Source: three-view drawing plus pictorial views. Frame: mm from the lowest corner of the part. Give positions to 0.01 mm unless a question says otherwise; leave off trailing zeros. Loops run counter-clockwise (first coordinate to the right, second up) from the corner with the lowest first, then second, coordinate; pieces in that order, holes last. Notation, with made-up numbers: M 41.25,-7 L 72.25,-7 A29 ccw 72.25,28 Z; hole C 29,-31 d2. An arc over 180 degrees is marked long. Answer as a JSON object with one key per item and string values. Group by question number.
1) Ray query, L1, parallel to X at y = 7, z = 147; L2, parallel to X at y = 18, z = 302 (1 decimal); L3, parallel to Z at x = 38.5, y = 15 (1 decimal). Return the intervals inside material, ascending.
2) Section query C-C on x = 79. Return loops of the section in (y, z).
3) Section query A-A on y = 14.5. Count the separate pieces of the cut face and the enclosed holes in it, plus the area to 3 significant figures.
4) First-contact query: P1, Ø9.5, axis at y = 13.5, z = 12.5, coming from the -X side; P2, Ø6, axis at x = 92.5, y = 11, coming from the -Z side; P3, Ø9.5, axis at y = 10, z = 10, coming from the +X side. Flat tips, straight axial feed; report the tip coordinate or a pass-through.
5) Section query B-B on z = 141. Return loops of the section in (x, y), plus the area to 3 significant figures.
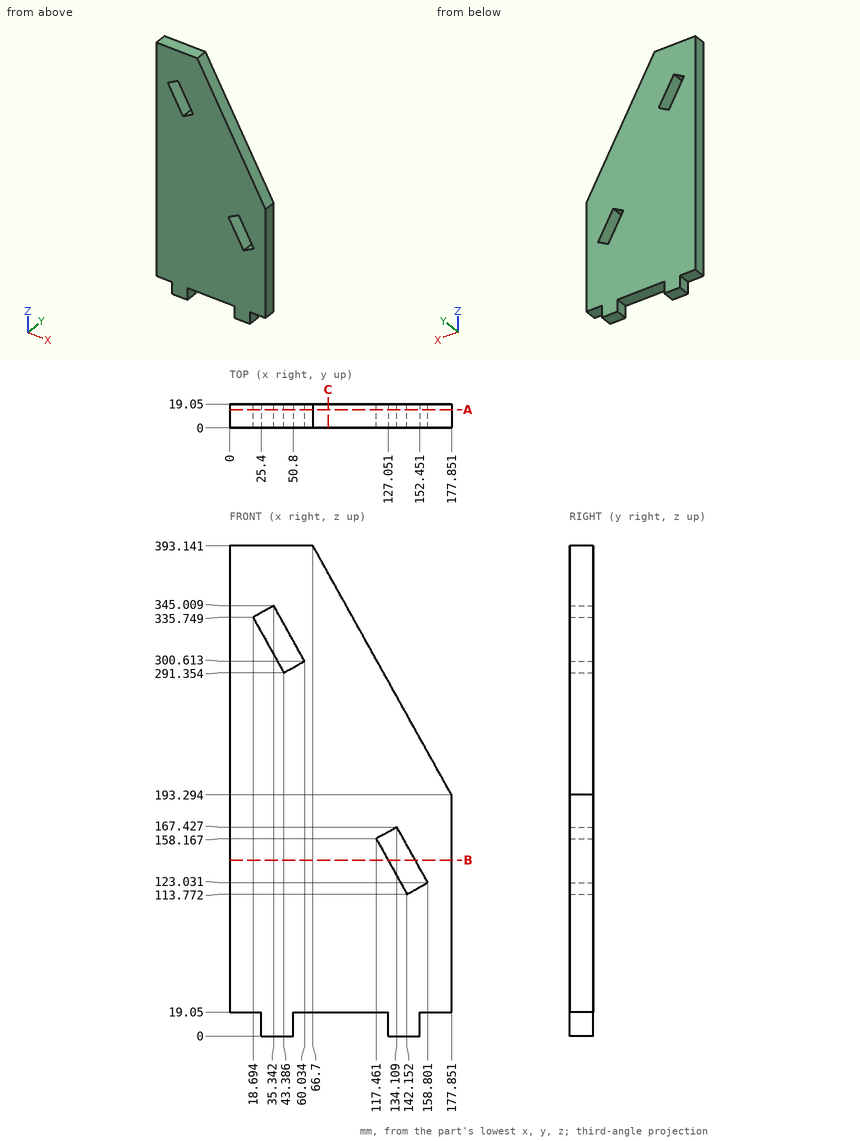
Output:
{
 "1": {"L1": "x = 0 to 123.67, 145.47 to 177.85", "L2": "x = 0 to 37.5, 59.3 to 117.4", "L3": "z = 0 to 300.1, 339.3 to 393.1"},
 "2": {"outline": "M 0,19.05 L 19.05,19.05 L 19.05,371.03 L 0,371.03 Z"},
 "3": {"separate pieces": "1", "enclosed holes": "2", "area": "54,500 mm^2"},
 "4": {"P1": "stops at x = 25.4", "P2": "stops at z = 19.05", "P3": "stops at x = 152.45"},
 "5": {"outline": "M 0,0 L 127.01,0 L 127.01,19.05 L 0,19.05 Z; M 148.81,0 L 177.85,0 L 177.85,19.05 L 148.81,19.05 Z", "area": "2,970 mm^2"}
}
